Autodesk Inventor part; units mm, degrees
ref_plane "YZ Plane" through (0, 0, 0) normal (1, 0, 0) x (0, 1, 0)
ref_plane "XZ Plane" through (0, 0, 0) normal (0, 1, 0) x (-1, 0, 0)
ref_plane "XY Plane" through (0, 0, 0) normal (0, 0, 1) x (1, 0, 0)
sketch "Skizze1" plane through (0, 0, 0) normal (0, 1, 0) x (-1, 0, 0)
  circle A0 centre (0, 0) radius 15
  dimension "d0" = 30
extrude "Extrusion1" add sketch "Skizze1" along normal blind 10
sketch "Skizze2" plane through (0, 0, 0) normal (0, -1, 0) x (1, 0, 0)
  line L0 (14.3188, 0.9) -> (12.9688, 0.9)
  line L1 (12.9688, -0.9) -> (14.3188, -0.9)
  line L2 (14.3188, -0.9) -> (14.3188, 0.9)
  line L3 (-21.3175, 0) -> (21.3175, 0)
  arc A0 (12.9688, 0.9) -> (0.9, 12.9688) centre (0, 0) ccw
  line L4 (-0.9, -12.9688) -> (-0.9, -14.3188)
  line L5 (-0.9, -14.3188) -> (0.9, -14.3188)
  line L6 (0.9, -14.3188) -> (0.9, -12.9688)
  line L7 (-12.9688, 0.9) -> (-14.3188, 0.9)
  line L8 (-14.3188, 0.9) -> (-14.3188, -0.9)
  line L9 (-14.3188, -0.9) -> (-12.9688, -0.9)
  line L10 (-0.9, 12.9688) -> (-0.9, 14.3188)
  line L11 (-0.9, 14.3188) -> (0.9, 14.3188)
  line L12 (0.9, 14.3188) -> (0.9, 12.9688)
  line L13 (0, -21.3175) -> (0, 21.3175)
  line L14 (-21.3175, 0) -> (21.3175, 0)
  arc A1 (0.9, -12.9688) -> (12.9688, -0.9) centre (0, 0) ccw
  arc A2 (-12.9688, -0.9) -> (-0.9, -12.9688) centre (0, 0) ccw
  arc A3 (-0.9, 12.9688) -> (-12.9688, 0.9) centre (0, 0) ccw
  circle A4 centre (0, 0) radius 4.2
  circle A5 centre (7, 7.1414) radius 1.2
  circle A6 centre (-5.6, -5.7131) radius 1.2
  dimension "d4" = 0.9
  dimension "d5" = 0.9
  dimension "d8" = 1.35
  dimension "d9" = 1.35
  dimension "d10" = 1.8
  dimension "d11" = 0.9
  dimension "d12" = 1.35
  dimension "d13" = 1.8
  dimension "d14" = 0.9
  dimension "d15" = 0.9
  dimension "d16" = 1.35
  dimension "d17" = 8.4
  dimension "d18" = 2.4
  dimension "d19" = 2.4
  dimension "d20" = 8
  dimension "d21" = 10
  dimension "d22" = 7
  dimension "d23" = 5.6
  dimension "d50" = 13
  dimension "d51" = 13
  dimension "d52" = 1.35
  dimension "d53" = 1.35
  dimension "d54" = 1.35
extrude "Extrusion2" cut sketch "Skizze2" against normal blind 3 contours L2 L3 A4 L13 L11 L12 A0 L0 | L2 L1 A1 L6 L5 L13 A4 L3 | A4 L3 L8 L7 A3 L10 L11 L13 | L13 L5 L4 A2 L9 L8 L3 A4
sketch "Skizze4" plane through (7, 0, 7.1414) normal (0, -1, 0) x (1, 0, 0)
  circle A0 centre (-7, -7.1414) radius 4.2
  circle A1 centre (-12.6, -12.8546) radius 1.2
  circle A2 centre (0, 0) radius 1.2
  line L0 (-7, -28.1414) -> (-7, 13.8586)
  dimension "d26" = 2.4
  dimension "d27" = 5.6
  dimension "d28" = 8
  dimension "d44" = 8.4
  dimension "d45" = 2.4
extrude "Extrusion3" add sketch "Skizze4" along normal blind 2
sketch "Skizze5" plane through (0, 10, 0) normal (0, 1, 0) x (1, 0, 0)
  circle A0 centre (0, 0) radius 19.262
  circle A1 centre (0, 0) radius 7
  dimension "d31" = 14
extrude "Extrusion4" cut sketch "Skizze5" against normal blind 7
fillet "Rundung1" radius 1 8 edges at (12.9688, 1.5, -0.9) (12.9688, 1.5, 0.9) (0.9, 1.5, -12.9688) (-0.9, 1.5, -12.9688) (-12.9688, 1.5, -0.9) (-12.9688, 1.5, 0.9) (-0.9, 1.5, 12.9688) (0.9, 1.5, 12.9688)
sketch "Skizze8" plane through (0, 10, 0) normal (0, 1, 0) x (1, 0, 0)
  circle A0 centre (0, 0) radius 1
  dimension "d46" = 2
extrude "Extrusion7" cut sketch "Skizze8" against normal blind 7
sketch "Skizze9" plane through (0, -2, 0) normal (0, -1, 0) x (1, 0, 0)
  line L0 (18.2687, 9.2162) -> (-7.478, -18.1772)
  line L1 (-7.478, -18.1772) -> (18.2687, -18.1772)
  line L2 (18.2687, -18.1772) -> (18.2687, 9.2162)
  line L3 (8.0673, 18.8043) -> (-17.6793, -8.5891)
  line L4 (-17.6793, -8.5891) -> (-17.6793, 18.8043)
  line L5 (-17.6793, 18.8043) -> (8.0673, 18.8043)
  point P0 (0, 0)
  dimension "d55" = 7
  dimension "d56" = 7
extrude "Extrusion8" cut sketch "Skizze9" against normal blind 50
sketch "Skizze10" plane through (0, -2, 0) normal (0, -1, 0) x (1, 0, 0)
  circle A0 centre (0, 0) radius 11.5
  circle A1 centre (0, 0) radius 18.9246
  dimension "d61" = 23
extrude "Extrusion9" cut sketch "Skizze10" against normal blind 10
sketch "Skizze11" plane through (0, -2, 0) normal (0, -1, 0) x (1, 0, 0)
  circle A0 centre (0, 0) radius 1
  circle A1 centre (0, 0) radius 4.2
extrude "Extrusion10" cut sketch "Skizze11" against normal blind 8.5 contours A0 | A1
sketch "Skizze13" plane through (0, 3, 0) normal (0, -1, 0) x (1, 0, 0)
  circle A0 centre (7, 7.1414) radius 1.2
  circle A1 centre (7, 7.1414) radius 1.2
  circle A2 centre (-5.6, -5.7131) radius 1.2
  circle A3 centre (-5.6, -5.7131) radius 1.2
  arc A4 (11.3495, 1.8544) -> (-0.5206, 11.4882) centre (0, 0) ccw
  line L0 (11.3495, 1.8544) -> (8.9749, -0.6721)
  line L1 (11.3495, 1.8544) -> (-1.1481, -11.4425)
  line L2 (-0.5206, 11.4882) -> (-11.4984, -0.1917)
  line L3 (1.2265, -8.916) -> (-1.1481, -11.4425)
  arc A5 (-11.4984, -0.1917) -> (-1.1481, -11.4425) centre (0, 0) ccw
  circle A6 centre (0, 0) radius 4.2
extrude "Extrusion11" add sketch "Skizze13" along normal blind 3.5
sketch "Skizze14" plane through (7, -2, 7.1414) normal (0, -1, 0) x (1, 0, 0)
  circle A0 centre (0, 0) radius 1.2
  circle A1 centre (0, 0) radius 1.2
  circle A2 centre (-12.6, -12.8546) radius 1.2
  circle A3 centre (-12.6, -12.8546) radius 1.2
  point P0 (-7, -7.1414)
extrude "Extrusion12" add sketch "Skizze14" along normal blind 0.5
sketch "Skizze15" plane through (0, 10, 0) normal (0, 1, 0) x (1, 0, 0)
  circle A0 centre (0, 0) radius 1
  circle A1 centre (0, 0) radius 2.35
  dimension "d68" = 4.7
extrude "Extrusion13" cut sketch "Skizze15" against normal blind 3.3 contours A0 | A1
sketch "Skizze17" plane through (0, -0.5, 0) normal (0, -1, 0) x (1, 0, 0)
  line L0 (1.2267, 11.8871) -> (-14.9812, -5.3574)
  line L1 (-0.5206, 11.4882) -> (-11.4984, -0.1917)
  line L2 (-14.9812, -5.3574) -> (-14.9812, 19.8141)
  line L3 (-14.9812, 19.8141) -> (1.2267, 11.8871)
  line L4 (-3.5303, -12.5169) -> (12.8557, 4.9171)
  line L5 (-1.1481, -11.4425) -> (5.1007, -4.7941)
  line L6 (12.8557, 4.9171) -> (12.8557, -12.5169)
  line L7 (12.8557, -12.5169) -> (-3.5303, -12.5169)
  point P0 (0, 0)
  point P1 (-5.1007, 4.7941)
  point P2 (-11.4984, -0.1917)
  dimension "d71" = 1
  dimension "d72" = 1
extrude "Extrusion14" cut sketch "Skizze17" against normal blind 15
properties part number "Adaptation_on_OPdevside_4_2"
For this review, take the finished solid that the model builds, in its own axes (mm). A direction names the side the tool comes from. Round coordinates to 2 decimals unless told otherwise and drop trailing zeros. Loops run counter-clockwise (first coordinate to the right, second up) from the corner with the lowest first, then second, coordinate; pieces in that order, holes last.
(1) Wall thickness on line 1 along X through (y, z) = (6.25, -0.25); line 2 along Z through (x, y) = (0, 5); line 3 along Z through (x, y) = (0, 7.6): over which ranges is each line inside the solid? List them lowest first.
Returned:
line 1: x = -7 to -4.19, 4.19 to 7
line 2: z = -7 to -4.2, 4.2 to 7
line 3: z = -7 to -2.35, 2.35 to 7
(2) We need section A-A (z = 0). Give the boundary of the cut face in (x, y).
Returned:
outline: (-9.95, -0.5) - (-4.2, -0.5) - (-4.2, 6.5) - (-1, 6.5) - (-1, 6.7) - (-2.35, 6.7) - (-2.35, 10) - (-7, 10) - (-7, 3) - (-9.95, 3) - close; (1, 6.5) - (4.2, 6.5) - (4.2, -0.5) - (8.23, -0.5) - (8.23, 3) - (7, 3) - (7, 10) - (2.35, 10) - (2.35, 6.7) - (1, 6.7) - close
(3) Clearance check with flat-ended pins moving along their axes: P1, Ø2.5, axis at x = -1, z = 0, coming from the +Y side; P2, Ø3, axis at x = -4, z = 4, coming from the -Y side; P3, Ø6, axis at y = 7.5, z = -5, coming from the -X side; P4, Ø2, axis at x = -5, z = 7.5, coming from the +Y side. State where each tip first meets the part, or that it passes through.
Returned:
P1: stops at y = 6.7
P2: stops at y = -0.5
P3: stops at x = -6.71
P4: passes through
(4) We need section B-B (y = 0.75). Give the boundary of the cut face in (x, z), plus the area to 3 significant figures.
Returned:
outline: (-11.4, -1.54) arc R11.5 ccw to (-2.35, -11.26) - (11.09, 3.04) arc R11.5 ccw to (0.83, 11.47) - close; hole circle Ø8.4 at (0, 0)
area: 231 mm2
(5) We need section D-D (x = -5.6). Give the boundary of the cut face in (y, z).
Returned:
outline: (-2.5, -6.91) - (-0.5, -6.91) - (-0.5, -10.04) - (3, -10.04) - (3, -4.2) - (10, -4.2) - (10, 4.2) - (3, 4.2) - (3, 4.62) - (-0.5, 4.62) - (-0.5, -4.51) - (-2.5, -4.51) - close
(6) Mouldability with a two-part tool opening along X and no side actions: class faces 1 (the flat face through (1, 6.5, -1)), 2 (the flat face through (-6, -2.5, -6)), 3 (the flat face through (4.278, 3.51, -4.209)), 4 (the cylindrical face through (-0.509, 8.373, 2.294)) as released by +X, released by -X, zero draft, split by the parting line, or undercut.
Returned:
face 1: undercut
face 2: zero draft
face 3: released by +X
face 4: undercut
(7) Tool access review of faces 5 (the flat face through (7, -2.5, 7)), 6 (the cylindrical face through (-5.27, 6.55, 4.61)), 7 (the cylindrical face through (6.74, -1.486, 8.313)): name each direction out of +Z, -Z, +X, -X, +Y, -Y from which nothing blocks a thin tool from reaching the whole face with its end or side.
Returned:
face 5: +Z, -Z, +X, -X, -Y
face 6: +Y
face 7: -Y
(8) We need section C-C (x = 0.5). Give the boundary of the cut face in (y, z).
Returned:
outline: (-0.5, -8.23) - (3, -8.23) - (3, -6.98) - (10, -6.98) - (10, -2.3) - (6.7, -2.3) - (6.7, -0.87) - (6.5, -0.87) - (6.5, -4.17) - (-0.5, -4.17) - close; (-0.5, 4.17) - (6.5, 4.17) - (6.5, 0.87) - (6.7, 0.87) - (6.7, 2.3) - (10, 2.3) - (10, 6.98) - (3, 6.98) - (3, 11.11) - (-0.5, 11.11) - close
